Check sheet for the modelled part. Datum: model origin and axes. Units: mm. A direction names the side the tool comes from. Coordinates: 2 decimals unless noted, no trailing zeros. Write each loop counter-clockwise with the first axis right and the second up, starting at its lowest first coordinate (ties: lowest second). Pieces come first, ordered by that corner, then holes. Notation, with made-up numbers: M 45.5,-34.5 L 99.5,-34.5 A11 cw 99.5,-28.5 Z; hole C 75.5,87.25 d4. An arc over 180 degrees is marked long. Answer as CSV lines item,"result".
Autodesk Inventor part; units mm, degrees
ref_plane "YZ Plane" through (0, 0, 0) normal (1, 0, 0) x (0, 1, 0)
ref_plane "XZ Plane" through (0, 0, 0) normal (0, 1, 0) x (-1, 0, 0)
ref_plane "XY Plane" through (0, 0, 0) normal (0, 0, 1) x (1, 0, 0)
sketch "スケッチ1" plane through (0, 0, 0) normal (1, 0, 0) x (0, 1, 0)
  line L0 (-20, 80) -> (20, 80)
  line L1 (20, 80) -> (20, -80)
  line L2 (20, -80) -> (-20, -80)
  line L3 (-20, -80) -> (-20, 80)
  point P0 (0, 0)
  dimension "d0" = 160
  dimension "d2" = 40
  dimension "d3" = 20
  dimension "d4" = 80
extrude "押し出し1" add sketch "スケッチ1" along normal blind 2
sketch "スケッチ2" plane through (2, 0, 0) normal (1, 0, 0) x (0, 0, -1)
  line L0 (80, -20) -> (80, 20)
  line L1 (80, 20) -> (-80, 20)
  line L2 (-80, 20) -> (80, 20)
  line L3 (80, 20) -> (80, 18)
  line L4 (80, 18) -> (-80, 18)
  line L5 (-80, 18) -> (-80, 20)
  point P0 (0, 0)
  dimension "d7" = 2
extrude "押し出し2" add sketch "スケッチ2" along normal blind 20
sketch "スケッチ3" plane through (0, 0, 0) normal (-1, 0, 0) x (0, 0, 1)
  line L0 (80, -20) -> (80, 20)
  line L1 (80, 20) -> (-80, 20)
  line L2 (-80, 20) -> (-80, -20)
  line L3 (-80, -20) -> (80, -20)
  line L4 (-60, -20) -> (-60, -8.0385)
  line L5 (-60, -8.0385) -> (-30, 0)
  line L6 (-30, 0) -> (80, 0)
  line L7 (80, 0) -> (80, 20)
  line L8 (-80, 6.6025) -> (-30, 20)
  point P0 (0, 0)
  dimension "d11" = 20
  dimension "d12" = 15
  dimension "d13" = 15
  dimension "d14" = 20
  dimension "d15" = 160
  dimension "d17" = 110
  dimension "d18" = 110
extrude "押し出し3" cut sketch "スケッチ3" against normal blind 20 contours L6 L5 L4 L3 L2 L8 L1 L0 keep common part
sketch "スケッチ6" plane through (0, 0, 0) normal (-1, 0, 0) x (0, 0, 1)
  line L0 (-60, -8.0385) -> (-60, -20)
  line L1 (-30, 0) -> (-60, -8.0385)
  line L2 (80, 0) -> (-30, 0)
  line L3 (80, 0) -> (80, 20)
  line L4 (80, 20) -> (-30, 20)
  line L5 (-80, 6.6025) -> (-30, 20)
  line L6 (-80, 6.6025) -> (-80, -20)
  line L7 (-80, -20) -> (-60, -20)
  arc A0 (-66, -16) -> (-74, -16) centre (-70, -16) ccw
  arc A1 (76, 14) -> (76, 6) centre (76, 10) ccw
  line L8 (-74, -16) -> (-74, -20)
  line L9 (-66, -16) -> (-66, -20)
  line L10 (76, 14) -> (80, 14)
  line L11 (76, 6) -> (80, 6)
  arc A2 (-60.8348, -20) -> (-60, -16) centre (-70, -16) ccw
  arc A3 (-80, -16) -> (-79.1652, -20) centre (-70, -16) ccw
  arc A4 (76, 0) -> (80, 0.8348) centre (76, 10) ccw
  arc A5 (80, 19.1652) -> (76, 20) centre (76, 10) ccw
  point P0 (0, 0)
  dimension "d37" = 8
  dimension "d39" = 8
  dimension "d40" = 4
  dimension "d41" = 4
  dimension "d42" = 10
  dimension "d43" = 10
extrude "押し出し6" cut sketch "スケッチ6" against normal blind 11 contours L0 A2 L7 L9 A0 L8 A3 L6 L5 L4 A5 L3 L10 A1 L11 A4 L2 L1 keep common part
sketch "スケッチ7" plane through (0, 0, 0) normal (-1, 0, 0) x (0, 0, 1)
  arc A0 (80, 19.1652) -> (76, 20) centre (76, 10) ccw
  arc A1 (-80, -16) -> (-79.1652, -20) centre (-70, -16) ccw
  line L0 (-79.1652, -20) -> (-74, -20)
  line L1 (80, 0.8348) -> (80, 6)
  circle A2 centre (76, 3) radius 1
  circle A3 centre (-77, -16) radius 1
  point P0 (0, 0)
  dimension "d46" = 2
  dimension "d48" = 7
  dimension "d49" = 4
  dimension "d50" = 4
  dimension "d51" = 7
hole "穴1" at (0, -16, -77) at (0, 3, 76) direction (1, 0, 0) diameter 2 end through all
pattern_circular "円形状パターン1" count 5 over 180 about axis through (0, -16, -70) along (1, 0, 0) of "穴1"
pattern_circular "円形状パターン2" count 5 over 180 about axis through (0, 10, 76) along (1, 0, 0) of "穴1"
sketch "スケッチ4" plane through (0, 20, -30) normal (0, 1, 0) x (1, 0, 0)
  line L0 (0, 0) -> (20, 0)
  line L1 (0, -110) -> (0, 0)
  line L2 (20, 0) -> (2, 0)
  line L3 (2, 0) -> (2, 8)
  line L4 (2, 8) -> (20, 8)
  line L5 (20, 8) -> (20, 0)
  line L6 (20, -110) -> (11, -110)
  line L7 (11, -110) -> (11, 0)
  line L8 (11, 0) -> (20, 0)
  line L9 (20, 0) -> (20, -110)
  line L10 (11, -110) -> (2, -110)
  line L11 (2, -110) -> (2, -20)
  line L12 (2, -20) -> (11, -20)
  line L13 (11, -20) -> (11, -110)
  line L14 (11, 0) -> (10, 0)
  line L15 (10, 0) -> (10, -20)
  line L16 (10, -20) -> (11, -20)
  line L17 (11, -20) -> (11, 0)
  point P0 (0, -30)
  dimension "d21" = 18
  dimension "d23" = 2
  dimension "d24" = 20
  dimension "d25" = 8
  dimension "d65" = 1
extrude "押し出し7" cut sketch "スケッチ4" against normal blind 2
sketch "スケッチ8" plane through (0, 20, 76) normal (0, 1, 0) x (1, 0, 0)
  line L0 (10, 86) -> (10, 106)
  line L1 (2, 106) -> (10, 106)
  circle A0 centre (5, 101) radius 1.3
  circle A1 centre (5, 91) radius 1.3
  point P0 (0, 76)
  dimension "d68" = 10
  dimension "d70" = 5
  dimension "d71" = 5
  dimension "d72" = 5
  dimension "d73" = 2.6
hole "穴2" at (5, 20, -15) at (5, 20, -25) direction (0, -1, 0) diameter 2.6 end through all
thread "ねじ3"
thread "ねじ4"
properties part number "09" material "アルミニウム 6061"
1) Section check A-A, the plane y = -4. Record the boundary of the cut face in (x, z).
Answer key:
outline,"M 0,-80 L 2,-80 L 2,-44.93 L 0,-44.93 Z"
2) Thickness scan on line 1 along Z through (x, y) = (5, 18.65); line 2 along Z through (x, y) = (0.7, -9); line 3 along Y through (x, z) = (0.5, 76). Record the ranges inside material, lowest first.
Answer key:
line 1,"z = -30 to -26.3, -23.7 to -16.3, -13.7 to -10"
line 2,"z = -80 to -71, -69 to -60"
line 3,"y = 0 to 2, 4 to 6, 14 to 16, 18 to 20"
3) Tool access check on faces 5 (the face through (1.6, 20, 0.2)), 6 (the face through (6, 18, -20)). Record the directions out of +Z, -Z, +X, -X, +Y, -Y that give a thin tool (end or side, any length) a straight path to the whole face; none if there is none.
Answer key:
face 5,"+Z, -Z, +X, -X, +Y"
face 6,"+Z, -Z, +X, -Y"
4) Section check B-B, the plane z = -54. Record the boundary of the cut face in (x, y).
Answer key:
outline,"M 0,-6.43 L 2,-6.43 L 2,13.57 L 0,13.57 Z"
5) Depth check by flat-ended pin: P1, Ø4, axis at x = 5, z = -15, coming from the +Y side; P2, Ø1.5, axis at x = 4, y = -13.5, coming from the +Z side; P3, Ø3, axis at y = 17, z = 76, coming from the +X side; P4, Ø2, axis at x = 1.5, z = 50.5, coming from the -Y side. Enter the tip coordinate at first touch or a pass-through.
Answer key:
P1,"stops at y = 20"
P2,"passes through"
P3,"stops at x = 2"
P4,"stops at y = 0"
6) Mould release check, pull along Z, two halves, no side actions. Record for faces 1 (the face through (0.986, 13.207, -55.35)), 2 (the face through (4.94, 18.99, -26.3)), 3 (the face through (0.986, -4.076, -45.21)), 4 (the face through (1, -12, -70)): pulls with the +Z half, pulls with the -Z half, needs draft (parallel to the pull), parting line crosses it, or undercut.
Answer key:
face 1,"pulls with the -Z half"
face 2,"undercut"
face 3,"pulls with the +Z half"
face 4,"undercut"
